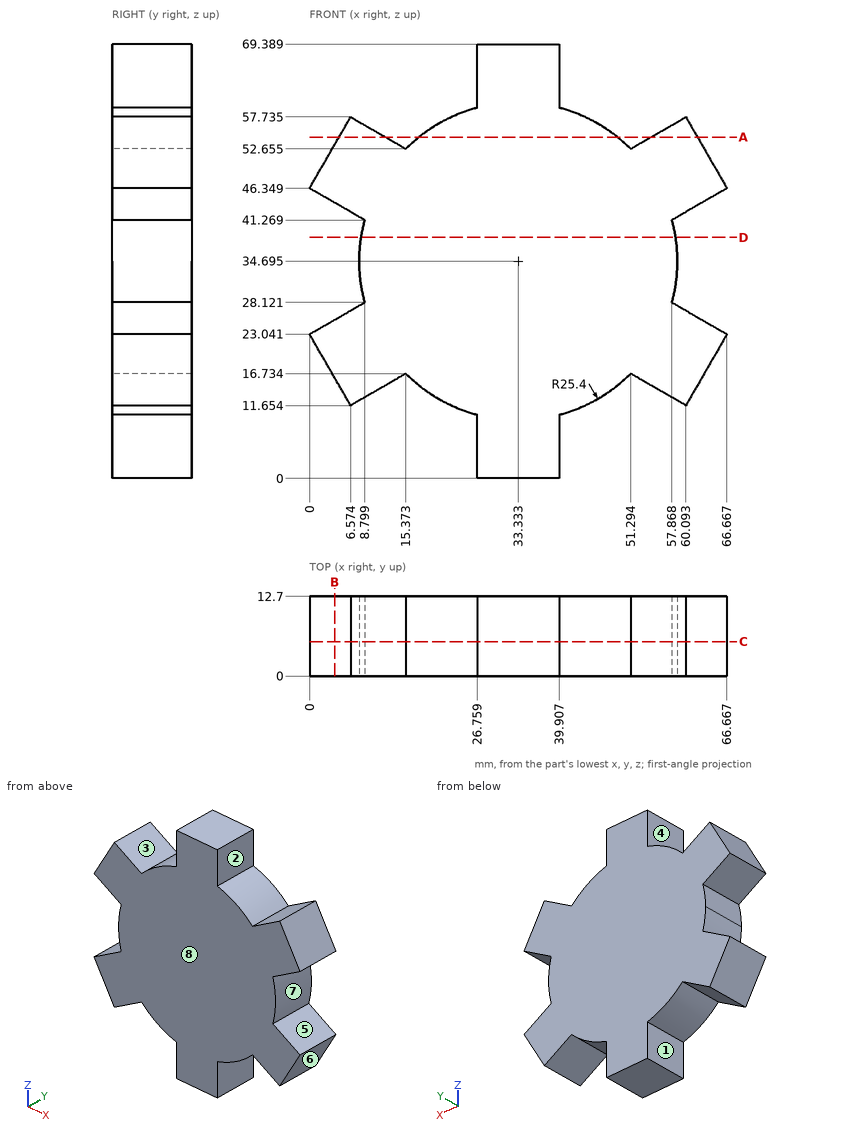
Design review of the part shown in the three views and the two pictorial views. Dimensions are in mm from the part's minimum x, y and z. A direction names the side the tool comes from. Round coordinates to 2 decimals unless told otherwise and drop trailing zeros. Write each loop counter-clockwise with the first axis right and the second up, starting at its lowest first coordinate (ties: lowest second). Pieces come first, ordered by that corner, then holes.
Item 1: For probe 1 along X at (y, z) = (3.5, 56) (1 decimal); probe 2 along X at (y, z) = (3, 6); probe 3 along Z at (x, y) = (64, 9.75) (1 decimal), list the stretches that pass through material, from the lowest coordinate up.
Item 2: The part is to be moulded in two halves that separate along Z. For the marked faces 5, 6, 7 and 8, say which applies: +Z half, -Z half, draft (parallel to the pull), parting line (faces both ways), or undercut.
Item 3: We need section A-A on z = 54.5. Write out the cut boundary in (x, y), and give its area (3 significant figures).
Item 4: We need section B-B on x = 4. Write out the cut boundary in (y, z), and give its area (3 significant figures).
Item 5: For the marked faces 1, 2, 3 and 4, list the 3-axis set-ups (+Z, -Z, +X, -X, +Y, -Y) from which the entire face can be reached by the end or side of a thin tool; tool diameter is ignored.
Item 6: We need section D-D on z = 38.5. Write out the cut boundary in (x, y), and give its area (3 significant figures).
Item 7: We need section C-C on y = 5.5. Write out the cut boundary in (x, z) (1 decimal).
Item 8: Clearance check with flat-ended pins moving along their axes: pin 1 Ø5 at (x, y) = (8, 3) entering from +Z (1 decimal); pin 2 Ø4 at (x, z) = (18, 27) entering from -Y; pin 3 Ø5 at (y, z) = (7.5, 63.5) entering from +X; pin 4 Ø2 at (x, z) = (7, 41) entering from -Y. State where each tip first meets the part, or that it passes through.
Returned:
1. probe 1: x = 5.6 to 9.6, 19.5 to 47.2, 57.1 to 61.1
1. probe 2: x = 26.76 to 39.91
1. probe 3: z = 18.4 to 24.6, 44.8 to 51
2. face 5: undercut
2. face 6: -Z half
2. face 7: undercut
2. face 8: draft
3. outline: (4.71, 0) - (12.18, 0) - (12.18, 12.7) - (4.71, 12.7) - close; (17.43, 0) - (49.24, 0) - (49.24, 12.7) - (17.43, 12.7) - close; (54.49, 0) - (61.96, 0) - (61.96, 12.7) - (54.49, 12.7) - close
3. area: 594 mm2
4. outline: (0, 16.11) - (12.7, 16.11) - (12.7, 25.35) - (0, 25.35) - close; (0, 44.04) - (12.7, 44.04) - (12.7, 53.28) - (0, 53.28) - close
4. area: 235 mm2
5. face 1: -Z, -X, +Y, -Y
5. face 2: +Z, +X, +Y, -Y
5. face 3: +Z, +Y, -Y
5. face 4: +Z, -X, +Y, -Y
6. outline: (8.22, 0) - (58.45, 0) - (58.45, 12.7) - (8.22, 12.7) - close
6. area: 638 mm2
7. outline: (0, 23) - (6.6, 11.7) - (15.4, 16.7) arc R25.4 ccw to (26.8, 10.2) - (26.8, 0) - (39.9, 0) - (39.9, 10.2) arc R25.4 ccw to (51.3, 16.7) - (60.1, 11.7) - (66.7, 23) - (57.9, 28.1) arc R25.4 ccw to (57.9, 41.3) - (66.7, 46.3) - (60.1, 57.7) - (51.3, 52.7) arc R25.4 ccw to (39.9, 59.2) - (39.9, 69.4) - (26.8, 69.4) - (26.8, 59.2) arc R25.4 ccw to (15.4, 52.7) - (6.6, 57.7) - (0, 46.3) - (8.8, 41.3) arc R25.4 ccw to (8.8, 28.1) - close
8. pin 1: stops at z = 57.7
8. pin 2: stops at y = 0
8. pin 3: stops at x = 39.91
8. pin 4: passes through
